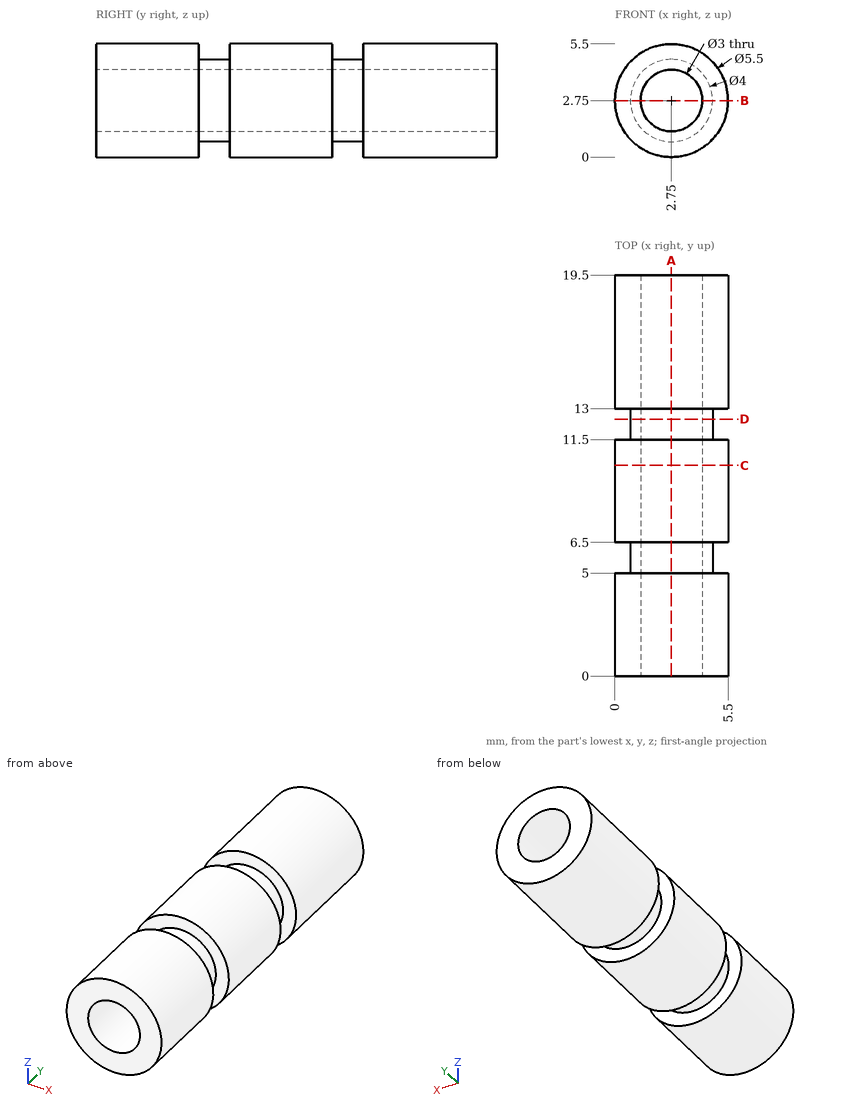
Could you check a few things on this drawing? It's one solid part, dimensions in mm from its lowest x, y, z. Give positions to 0.01 mm unless a question says otherwise; leave off trailing zeros. Loops run counter-clockwise (first coordinate to the right, second up) from the corner with the lowest first, then second, coordinate; pieces in that order, holes last. Notation, with made-up numbers: M 48.25,-38 L 60.25,-38 A12 cw 60.25,-20 Z; hole C -14.5,-19 d4. An arc over 180 degrees is marked long. Answer as a JSON object with one key per item and string values.
Q1. Suppose I cut it at C-C, the plane y = 10.25. List the corners of the cut face in (x, z) for me.
Values found:
{"outline": "C 2.75,2.75 d5.5; hole C 2.75,2.75 d3"}
Q2. Suppose I cut it at D-D, the plane y = 12.5. List the corners of the cut face in (x, z) for me.
Values found:
{"outline": "C 2.75,2.75 d4; hole C 2.75,2.75 d3"}
Q3. Suppose I cut it at B-B, the plane z = 2.75. List the corners of the cut face in (x, y) for me.
Values found:
{"outline": "M 0,0 L 1.25,0 L 1.25,19.5 L 0,19.5 L 0,13 L 0.75,13 L 0.75,11.5 L 0,11.5 L 0,6.5 L 0.75,6.5 L 0.75,5 L 0,5 Z; M 4.25,0 L 5.5,0 L 5.5,5 L 4.75,5 L 4.75,6.5 L 5.5,6.5 L 5.5,11.5 L 4.75,11.5 L 4.75,13 L 5.5,13 L 5.5,19.5 L 4.25,19.5 Z"}
Q4. If I drill on probe 1 along Y at (x, z) = (0.75, 3.35); probe 2 along X at (y, z) = (7.5, 2.75); probe 3 along X at (y, z) = (5.7, 2.75), over which ranges is the centre line in solid material (lowest first)? Write a range as [from, to].
Values found:
{"probe 1": "y = [0, 5], [6.5, 11.5], [13, 19.5]", "probe 2": "x = [0, 1.25], [4.25, 5.5]", "probe 3": "x = [0.75, 1.25], [4.25, 4.75]"}
Q5. For P1, Ø2.5, axis at x = 2.75, z = 2.75, coming from the -Y side; P2, Ø3, axis at x = 1.5, z = 3, coming from the -Y side, each with a flat end and sliding along its axis, tell me the tip position at first contact or that it passes through.
Values found:
{"P1": "passes through", "P2": "stops at y = 0"}
Q6. Suppose I cut it at A-A, the plane x = 2.75. List the corners of the cut face in (y, z) for me.
Values found:
{"outline": "M 0,0 L 5,0 L 5,0.75 L 6.5,0.75 L 6.5,0 L 11.5,0 L 11.5,0.75 L 13,0.75 L 13,0 L 19.5,0 L 19.5,1.25 L 0,1.25 Z; M 0,4.25 L 19.5,4.25 L 19.5,5.5 L 13,5.5 L 13,4.75 L 11.5,4.75 L 11.5,5.5 L 6.5,5.5 L 6.5,4.75 L 5,4.75 L 5,5.5 L 0,5.5 Z"}
